For this review, take the finished solid that the model builds, in its own axes (mm). Face numbers are marked on the shaded views. A direction names the side the tool comes from. Give positions to 0.01 mm unless a question says otherwise; leave off trailing zeros. Order: outer loops, then holes, each group sorted by start corner. A loop starts at its lowest first (then second) coordinate and runs counter-clockwise, first axis right, second up. Notation, with made-up numbers: (76.25, 10.5) - (130.25, 10.5) arc R12 cw to (130.25, 32.5) - close; hole circle Ø7 at (33.25, -21.75). An arc over 180 degrees is marked (long way). One line per item, written item: value.
Autodesk Inventor part; units mm, degrees
ref_plane "YZ Plane" through (0, 0, 0) normal (1, 0, 0) x (0, 1, 0)
ref_plane "XZ Plane" through (0, 0, 0) normal (0, 1, 0) x (-1, 0, 0)
ref_plane "XY Plane" through (0, 0, 0) normal (0, 0, 1) x (1, 0, 0)
sketch "スケッチ1" plane through (0, 0, 0) normal (0, 0, 1) x (1, 0, 0)
  line L0 (-4, -7) -> (0, -7)
  line L1 (4, -3) -> (4, 0)
  arc A0 (-4, -7) -> (-4, -9) centre (-4, -8) ccw
  line L2 (-4, -9) -> (-4, -12)
  arc A1 (-5.5, 0) -> (-2.5, 0) centre (-4, 0) ccw
  arc A2 (-7.9856, -8.3391) -> (-4, -12) centre (-4, -8) ccw
  line L3 (-7.9856, -8.3391) -> (-8.3056, -4.5778)
  line L4 (-8.5, 0) -> (-5.5, 0)
  line L5 (-1, 0) -> (-1, -3)
  line L6 (2, -3) -> (2, 0)
  line L7 (-2.5, 0) -> (-1, 0)
  line L8 (2, 0) -> (4, 0)
  arc A3 (-1, -3) -> (2, -3) centre (0.5, -3) ccw
  circle A4 centre (-4, 0) radius 5 construction
  line L9 (-9, 0) -> (-9, -7) construction
  arc A5 (-8.5, 0) -> (-8.3056, -4.5778) centre (45.5, 0) ccw
  circle A6 centre (-4, 0) radius 3 construction
  arc A7 (0, -7) -> (4, -3) centre (0, -3) ccw
  point P0 (0, 0)
  point P1 (0, 0)
  point P2 (0, 0)
  dimension "d14" = 10
  dimension "d17" = 6
  dimension "d3" = 1
  dimension "d4" = 3
  dimension "d6" = 3
  dimension "d8" = 4
  dimension "d11" = 3
  dimension "d13" = 2
  dimension "d15" = 5
  dimension "d16" = 54
  dimension "d31" = 4
  dimension "d32" = 7
  dimension "d41" = 4
  dimension "d42" = 4
  dimension "d43" = 4
  dimension "d46" = 1.5
  dimension "d47" = 3
  dimension "d48" = 3
  dimension "d53" = 0
extrude "押し出し1" add sketch "スケッチ1" along normal blind 3
mirror "ミラー1" about plane through (-1, 0, 0) normal (0, 1, 0) of "押し出し1"
chamfer "面取り1" distance 1.5 angle 45 1 edges at (-4, -1.5, 3)
properties part number "ShaftBase2"
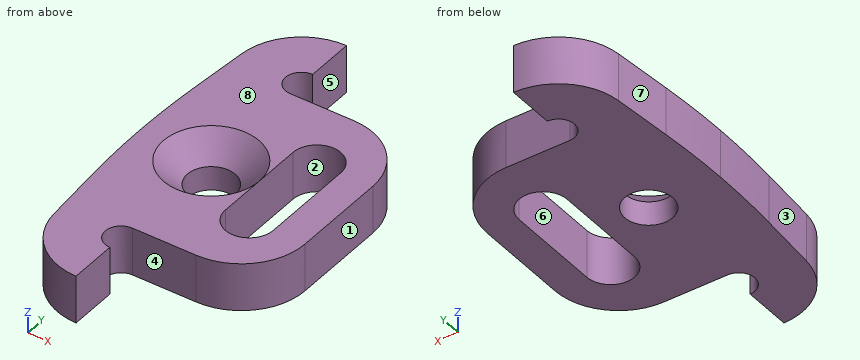
(1) Machinability: for the marked faces 4, 5, 6, 7 and 8, which of the approach directions +Z, -Z, +X, -X, +Y, -Y give a long, thin tool a straight path to every point of the face, cutting with its end or side? Answer none if there is none.
Answers below:
face 4: +Z, -Z, +X, -Y
face 5: +Z, -Z, +X, +Y
face 6: +Z, -Z
face 7: +Z, -Z, -X, +Y
face 8: +Z, +X, -X, +Y, -Y
(2) Take a section at D-D (y = -7.5). Write out the cut boundary in (x, z), then the cut area to 3 significant figures.
Answers below:
outline: (-8.06, 0) - (-4.87, 0) - (-4.87, 3) - (-8.06, 3) - close
area: 9.57 mm^2
(3) Wall thickness on line 1 (X direction, y = 0, z = 0.45); line 2 (Y direction, x = -4.75, z = 2.35); line 3 (X direction, y = 3.25, z = 1.4): over which ranges is each line inside the solid? List them lowest first. Write a range as from..to.
Answers below:
line 1: x = -8.5..-5.5, -2.5..-1, 2..4
line 2: y = -11.93..-8.66, -7.34..-2.23, 2.23..7.34, 8.66..11.93
line 3: x = -8.4..-0.98, 1.98..3.99
(4) Take a section at C-C (y = 3.25). Write out the cut boundary in (x, z), then the cut area to 3 significant figures.
Answers below:
outline: (-8.4, 0) - (-0.98, 0) - (-0.98, 3) - (-8.4, 3) - close; (1.98, 0) - (3.99, 0) - (3.99, 3) - (1.98, 3) - close
area: 28.3 mm^2
(5) Take a section at B-B (x = 0.25). Write out the cut boundary in (y, z), then the cut area to 3 significant figures.
Answers below:
outline: (-6.99, 0) - (-4.48, 0) - (-4.48, 3) - (-6.99, 3) - close; (4.48, 0) - (6.99, 0) - (6.99, 3) - (4.48, 3) - close
area: 15.1 mm^2
(6) For P1, Ø5, axis at x = -4, y = 0, coming from the -Z side; P2, Ø0.9, axis at y = 10, z = 2, coming from the +X side; P3, Ø1, axis at x = -1, z = 0.5, coming from the -Y side, all flat-tipped, find the tip position at first contact; note any pin that passes through.
Answers below:
P1: stops at z = 0
P2: stops at x = -4
P3: stops at y = -7
(7) Draft analysis for pull direction X (two halves, no side actions). For the marked faces 1, 2 and 3, state which applies: pulls with the +X half, pulls with the -X half, needs draft (parallel to the pull), parting line crosses it, or undercut.
Answers below:
face 1: pulls with the +X half
face 2: undercut
face 3: pulls with the -X half
(8) Take a section at A-A (z = 1.15). Write out the cut boundary in (x, y), then the cut area to 3 significant figures.
Answers below:
outline: (-8.5, 0) arc R53.99 ccw to (-8.31, -4.58) - (-7.99, -8.34) arc R4 ccw to (-4, -12) - (-4, -9) arc R1 cw to (-4, -7) - (0, -7) arc R4 ccw to (4, -3) - (4, 3) arc R4 ccw to (0, 7) - (-4, 7) arc R1 cw to (-4, 9) - (-4, 12) arc R4 ccw to (-7.99, 8.34) - (-8.31, 4.58) arc R53.99 ccw to start; hole circle Ø3 at (-4, 0); hole (-1, -3) arc R1.5 ccw to (2, -3) - (2, 3) arc R1.5 ccw to (-1, 3) - close
area: 164 mm^2
